Can you work these out from the model? Positions are in its coordinate system, mm. A direction names the side the tool comes from. Round coordinates to 2 decimals unless told otherwise and drop trailing zeros. Order: outer loops, then holes, each group sorted by start corner. A loop starts at its lowest first (then second) coordinate and runs counter-clockwise, first axis right, second up. Notation, with made-up numbers: M 54,85.25 L 99,85.25 A14 ccw 99,99.25 Z; hole C 75.5,-12.5 d6. An arc over 180 degrees is marked long. Answer as a JSON object with one key per item and string values. Group by question number.
from build123d import *

# Parameters (mm, degrees)
F0_W     = 362.9276417196
F0_H     = 246.9854429364
F1_DEPTH = 25
F2_T     = -2.5
F3_W     = 357.9549430311
F3_H     = 45.3172796965
F4_DEPTH = 25
F6_DEPTH = 407
F8_DEPTH = 21.2


with BuildPart() as f1:
    # F0 (on Front) → F1 (new body)
    with BuildSketch(Plane.XZ):
        with Locations((197.4523235112, -37.3292528093)):
            Rectangle(F0_W, F0_H)
    extrude(amount=F1_DEPTH)

    # F2
    f2_openings = [f1.faces().sort_by_distance(p)[0] for p in [
        (197.452324, -25, -37.329253),
    ]]
    offset(amount=F2_T, openings=f2_openings)

    # F3 (on face) → F4 (cut)
    with BuildSketch(Plane.XZ.offset(25)):
        with Locations((197.465974167, -180.9806141257)):
            Rectangle(F3_W, F3_H)
    extrude(amount=-F4_DEPTH, mode=Mode.SUBTRACT)

    # F5 (on face) → F6 (cut)
    with BuildSketch(Plane.YZ.offset(378.916144371)):
        with BuildLine():
            Line((-11.0355205834, 31.4804576337), (-25, 31.4804576337))
            Line((-25, 31.4804576337), (-25, 25.6381239742))
            Line((-25, 25.6381239742), (-11.0355205834, 25.6381239742))
            Line((-11.0355205834, 25.6381239742), (-11.0355205834, 10.0848458931))
            ThreePointArc((-11.0355205834, 10.0848458931), (-10.7426273646, 9.3777391119), (-10.0355205834, 9.0848458931))
            Line((-10.0355205834, 9.0848458931), (-6.8423313312, 9.0848458931))
            ThreePointArc((-6.8423313312, 9.0848458931), (-6.13522455, 9.3777391119), (-5.8423313312, 10.0848458931))
            Line((-5.8423313312, 10.0848458931), (-5.8423313312, 47.0337403715))
            ThreePointArc((-5.8423313312, 47.0337403715), (-6.13522455, 47.7408471527), (-6.8423313312, 48.0337403715))
            Line((-6.8423313312, 48.0337403715), (-10.0355205834, 48.0337403715))
            ThreePointArc((-10.0355205834, 48.0337403715), (-10.7426273646, 47.7408471527), (-11.0355205834, 47.0337403715))
            Line((-11.0355205834, 47.0337403715), (-11.0355205834, 31.4804576337))
        make_face()
        with BuildLine():
            Line((-11.0355205834, -127.2254977375), (-25, -127.2254977375))
            Line((-25, -127.2254977375), (-25, -133.0678313971))
            Line((-25, -133.0678313971), (-11.0355205834, -133.0678313971))
            Line((-11.0355205834, -133.0678313971), (-11.0355205834, -148.6211094782))
            ThreePointArc((-11.0355205834, -148.6211094782), (-10.7426273646, -149.3282162594), (-10.0355205834, -149.6211094782))
            Line((-10.0355205834, -149.6211094782), (-6.8423313312, -149.6211094782))
            ThreePointArc((-6.8423313312, -149.6211094782), (-6.13522455, -149.3282162594), (-5.8423313312, -148.6211094782))
            Line((-5.8423313312, -148.6211094782), (-5.8423313312, -111.6722149998))
            ThreePointArc((-5.8423313312, -111.6722149998), (-6.13522455, -110.9651082186), (-6.8423313312, -110.6722149998))
            Line((-6.8423313312, -110.6722149998), (-10.0355205834, -110.6722149998))
            ThreePointArc((-10.0355205834, -110.6722149998), (-10.7426273646, -110.9651082186), (-11.0355205834, -111.6722149998))
            Line((-11.0355205834, -111.6722149998), (-11.0355205834, -127.2254977375))
        make_face()
    extrude(amount=-F6_DEPTH, mode=Mode.SUBTRACT)

    # F7 (on face) → F8 (cut)
    with BuildSketch(Plane.XZ.offset(25)):
        Polygon((367.0578853405, 86.1634686589), (370.9844340809, 83.6634686589), (376.416144371, 83.6634686589), (376.416144371, 80.2051451735), (378.916144371, 78.6134165555), (378.916144371, 86.1634686589), align=None)
        Polygon((15.9885026515, 80.7326063961), (16.7155197178, 77.799282968), (18.4885026515, 79.6139837289), (18.4885026515, 83.6634686589), (22.4448947056, 83.6634686589), (24.8874226582, 86.1634686589), (15.9885026515, 86.1634686589), align=None)
    extrude(amount=-F8_DEPTH, mode=Mode.SUBTRACT)


solid = f1.part
Item 1: Suppose I cut it at A-A, the plane z = 20.5. Write out the boundary of the cut face in (x, y), and give its area (3 significant figures).
Item 2: I need wall thicknesses on line 1 (X direction, y = -18.25, z = -51.5); line 2 (Y direction, x = 210, z = -3); line 3 (Z direction, x = 343, y = -18.5). Which ranges of each line are inside material? Lowest first, please.
Item 3: Suppose I cut it at C-C, the plane z = -19. Write out the boundary of the cut face in (x, y), and give its area (3 significant figures).
Item 4: Suppose I cut it at B-B, the plane x = 145.5. Write out the boundary of the cut face in (y, z), and give its area (3 significant figures).
Item 5: On a 3-axis mill with a long thin cutter (end or side, diameter ignored), from which of +Z, -Z, +X, -X, +Y, -Y can I reach the whole of each face in a straight line? I mean faces 1 (the face through (19, -3.8, 84)), 2 (the face through (376.416, -14, -39)), 3 (the face through (197, -1, -158.322)), 4 (the face through (376, -3.8, 84)), 5 (the face through (195, 0, -36)). Say none if no direction works.
Item 6: I'm going to push flat-ended pins straight in: pin 1 Ø10 at (x, z) = (253.5, 8.5) entering from -Y; pin 2 Ø3 at (x, y) = (378, -9) entering from +Z; pin 3 Ø0.8 at (x, y) = (378, -8.5) entering from +Z. Where does each tip first touch, or does it pass through?
Computed:
{
 "1": {"outline": "M 15.99,-25 L 18.49,-25 L 18.49,-11.04 L 15.99,-11.04 Z; M 15.99,-5.84 L 18.49,-5.84 L 18.49,-2.5 L 376.42,-2.5 L 376.42,-5.84 L 378.92,-5.84 L 378.92,0 L 15.99,0 Z; M 376.42,-25 L 378.92,-25 L 378.92,-11.04 L 376.42,-11.04 Z", "area": "994 mm^2"},
 "2": {"line 1": "x = 15.99 to 18.49, 376.42 to 378.92", "line 2": "y = -2.5 to 0", "line 3": "z = 83.66 to 86.16"},
 "3": {"outline": "M 15.99,-25 L 18.49,-25 L 18.49,-2.5 L 376.42,-2.5 L 376.42,-25 L 378.92,-25 L 378.92,0 L 15.99,0 Z", "area": "1,020 mm^2"},
 "4": {"outline": "M -25,83.66 L -2.5,83.66 L -2.5,-158.32 L 0,-158.32 L 0,86.16 L -25,86.16 Z", "area": "667 mm^2"},
 "5": {"face 1": "+Z, -Y", "face 2": "-Z, -Y", "face 3": "-Z, +Y, -Y", "face 4": "+Z, +X, -Y", "face 5": "+Z, -Z, +X, -X, +Y"},
 "6": {"pin 1": "stops at y = -2.5", "pin 2": "stops at z = 80.15", "pin 3": "stops at z = 79.45"}
}
